Source: CAD feature listing. Evaluate the final solid. Frame: model axes, mm. A direction names the side the tool comes from. Give positions to 0.01 mm unless a question says otherwise; leave off trailing zeros. Loops run counter-clockwise (first coordinate to the right, second up) from the corner with the lowest first, then second, coordinate; pieces in that order, holes last. Notation, with made-up numbers: (-26, -28) - (21, -28) arc R10 ccw to (21, -16) - close; hole circle Ø2 at (46.5, 28). An arc over 180 degrees is marked (long way). Put each result on its own line as item: value.
```python
from build123d import *

# Parameters (mm, degrees)
MAIN_BLOCK_EXTRUDE_DEPTH = 65.09
SHELL1_T                 = -5
SLANT_DEPTH              = 405.38


with BuildPart() as part:
    # Sketch1 → Main block extrude (new, symmetric)
    with BuildSketch(Plane(origin=(0, 0, 0), x_dir=(1, 0, 0), z_dir=(0, 1, 0))):
        Polygon((0, 0), (-71.265, -399.066716446), (71.265, -399.066716446), align=None)
    extrude(amount=MAIN_BLOCK_EXTRUDE_DEPTH, both=True)

    # Shell1
    shell1_openings = [part.faces().sort_by_distance(p)[0] for p in [
        (0, -65.09, 266.044477631),
    ]]
    offset(amount=SHELL1_T, openings=shell1_openings, kind=Kind.INTERSECTION)

    # Sketch2 → Slant (add)
    with BuildSketch(Plane(origin=(71.265, 0, 399.066716446), x_dir=(0, -1, 0), z_dir=(0.17579801667571168, 0, 0.9844262579456555))):
        Polygon((-65.09, 0), (65.09, 0), (-65.09, 8.560443406), align=None)
    extrude(amount=-SLANT_DEPTH)


solid = part.part
```
1) Material intervals for line 1 along Y through (x, z) = (-10.5, 260); line 2 along X through (y, z) = (-60, 29); line 3 along X through (y, z) = (-36, 366.5), sorted ascending. Write a range as [from, to].
Check result:
line 1: [60.09, 65.09]
line 2: [-5.18, -0.1], [0.1, 5.52]
line 3: [-65.45, -60.37], [60.37, 67.39]
2) Section query A-A, the plane y = 39.5. Output: boundary loops of the cut face in (x, z) (3 decimals).
Check result:
outline: (-71.265, 399.067) - (0, 0) - (6.771, -1.209) - (78.036, 397.858) - (71.265, 399.067) - close; hole (-65.293, 394.067) - (0, 28.442) - (65.293, 394.067) - close
3) Section query B-B, the plane z = 324. Output: boundary loops of the cut face in (x, y), plus the area to 3 significant figures.
Check result:
outline: (-57.86, -65.09) - (-52.78, -65.09) - (-52.78, 60.09) - (52.78, 60.09) - (52.78, -65.09) - (57.86, -65.09) - (66.56, 65.09) - (-57.86, 65.09) - close
area: 2,420 mm²
4) Access query for faces 5 (the flat face through (73.66, 29.84, 398.64)), 6 (the flat face through (33.1, -1.6, 213.8)). Directions: +Z, -Z, +X, -X, +Y, -Y. A direction counts if a zero-diameter tool reaches every point of the face in a straight line with its end or side. Return the directions, or none.
Check result:
face 5: +Z, +X, +Y, -Y
face 6: -Y
5) Section query D-D, the plane y = 23.5. Output: boundary loops of the cut face in (x, z) (3 decimals).
Check result:
outline: (-71.265, 399.067) - (0, 0) - (5.735, -1.024) - (77, 398.043) - (71.265, 399.067) - close; hole (-65.293, 394.067) - (0, 28.442) - (65.293, 394.067) - close
6) Mould query, pull axis Z, two halves, no side actions, for faces 1 (the flat face through (-1, 60.09, 249)), 2 (the flat face through (2.4, 29.84, -0.43)), 3 (the flat face through (-1, 1, 399.067)), 4 (the flat face through (31, -65.09, 199)). Classes: pulls with the +Z half, pulls with the -Z half, needs draft (parallel to the pull), parting line crosses it, or undercut.
Check result:
face 1: undercut
face 2: pulls with the -Z half
face 3: pulls with the +Z half
face 4: needs draft
7) Pin query (flat end, axial travel): P1, Ø5, axis at y = -6.5, z = 230.5, coming from the -X side. Return the tip coordinate at first contact, or that it passes through.
Check result:
P1: x = -41.61
8) Section query C-C, the plane x = 46.5. Output: boundary loops of the cut face in (y, z), plus the area to 3 significant figures.
Check result:
outline: (-65.09, 260.39) - (65.09, 211.69) - (65.09, 399.07) - (-65.09, 399.07) - (-65.09, 394.07) - (60.09, 394.07) - (60.09, 288.83) - (-65.09, 288.83) - close
area: 8,050 mm²
